Can you work these out from the model? Positions are in its coordinate system, mm. Round coordinates to 2 decimals unless told otherwise and drop trailing zeros. Loops run counter-clockwise (first coordinate to the right, second up) from the corner with the lowest first, then second, coordinate; pieces in that order, holes last.
(1) I want a section at B-B on y = 152.4. Write out the boundary of the cut face in (x, z).
(2) Will this pin go through, and if not, where does the flat tip stop? pin 1 Ø7 at (y, z) = (152.4, 69.85) entering from +X.
(3) I want a section at A-A on z = -139.7. Write out the boundary of the cut face in (x, y) (1 decimal).
(4) If I drill on line 1 along Y through (x, z) = (1.1, 69.85) (3 decimals); line 2 along Y through (x, z) = (3.85, 69) (3 decimals); line 3 along Z through (x, y) = (1.4, -152), over which ranges is the centre line in solid material (lowest first)?
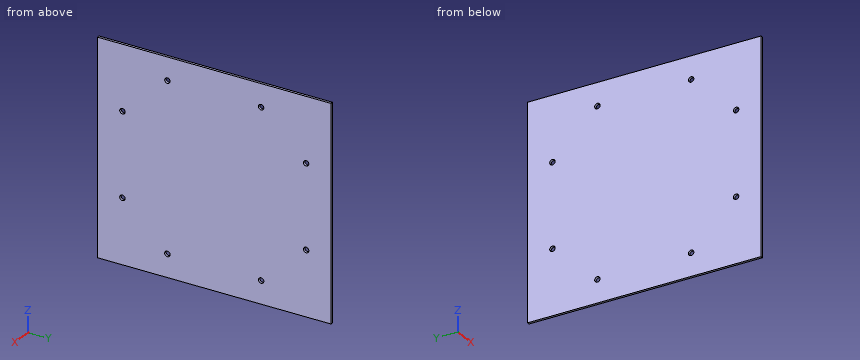
from build123d import *

# Parameters (mm, degrees)
SKETCH1_W            = 355.6
SKETCH1_H            = 387.35
SKETCH1_R            = 4.0005
BOSS_EXTRUDE1_DEPTH  = 4.064
M8_CLEARANCE_HOLE1_D = 9


with BuildPart() as part:
    # Sketch1 → Boss-Extrude1 (new body)
    # profile 1 of 9: a face of its own
    with BuildSketch(Plane(origin=(0, 0, 0), x_dir=(0, 0, -1), z_dir=(1, 0, 0))):
        Rectangle(SKETCH1_W, SKETCH1_H)
        with Locations((139.7, 77.7875)):
            Circle(SKETCH1_R, mode=Mode.SUBTRACT)
        with Locations((69.85, 152.4)):
            Circle(SKETCH1_R, mode=Mode.SUBTRACT)
        with Locations((-139.7, 77.7875)):
            Circle(SKETCH1_R, mode=Mode.SUBTRACT)
        with Locations((-139.7, -77.7875)):
            Circle(SKETCH1_R, mode=Mode.SUBTRACT)
        with Locations((-69.85, -152.4)):
            Circle(SKETCH1_R, mode=Mode.SUBTRACT)
        with Locations((69.85, -152.4)):
            Circle(SKETCH1_R, mode=Mode.SUBTRACT)
        with Locations((-69.85, 152.4)):
            Circle(SKETCH1_R, mode=Mode.SUBTRACT)
        with Locations((139.7, -77.7875)):
            Circle(SKETCH1_R, mode=Mode.SUBTRACT)
    # profile 2 of 9: a face of its own
    with BuildSketch(Plane(origin=(0, 0, 0), x_dir=(0, 0, -1), z_dir=(1, 0, 0))):
        with Locations((-69.85, -152.4)):
            Circle(SKETCH1_R)
    # profile 3 of 9: a face of its own
    with BuildSketch(Plane(origin=(0, 0, 0), x_dir=(0, 0, -1), z_dir=(1, 0, 0))):
        with Locations((69.85, -152.4)):
            Circle(SKETCH1_R)
    # profile 4 of 9: a face of its own
    with BuildSketch(Plane(origin=(0, 0, 0), x_dir=(0, 0, -1), z_dir=(1, 0, 0))):
        with Locations((139.7, -77.7875)):
            Circle(SKETCH1_R)
    # profile 5 of 9: a face of its own
    with BuildSketch(Plane(origin=(0, 0, 0), x_dir=(0, 0, -1), z_dir=(1, 0, 0))):
        with Locations((139.7, 77.7875)):
            Circle(SKETCH1_R)
    # profile 6 of 9: a face of its own
    with BuildSketch(Plane(origin=(0, 0, 0), x_dir=(0, 0, -1), z_dir=(1, 0, 0))):
        with Locations((69.85, 152.4)):
            Circle(SKETCH1_R)
    # profile 7 of 9: a face of its own
    with BuildSketch(Plane(origin=(0, 0, 0), x_dir=(0, 0, -1), z_dir=(1, 0, 0))):
        with Locations((-69.85, 152.4)):
            Circle(SKETCH1_R)
    # profile 8 of 9: a face of its own
    with BuildSketch(Plane(origin=(0, 0, 0), x_dir=(0, 0, -1), z_dir=(1, 0, 0))):
        with Locations((-139.7, 77.7875)):
            Circle(SKETCH1_R)
    # profile 9 of 9: a face of its own
    with BuildSketch(Plane(origin=(0, 0, 0), x_dir=(0, 0, -1), z_dir=(1, 0, 0))):
        with Locations((-139.7, -77.7875)):
            Circle(SKETCH1_R)
    extrude(amount=BOSS_EXTRUDE1_DEPTH)

    # M8 Clearance Hole1 (through all)
    with Locations(Plane(origin=(4.064, 0, 0), x_dir=(0, 0, -1), z_dir=(1, 0, 0))):
        with Locations((-139.7, 77.7875), (-69.85, 152.4), (69.85, 152.4), (139.7, 77.7875), (139.7, -77.7875), (69.85, -152.4), (-69.85, -152.4), (-139.7, -77.7875)):
            Hole(M8_CLEARANCE_HOLE1_D / 2)


solid = part.part
Filled sheet:
1. outline: (0, -177.8) - (4.06, -177.8) - (4.06, -74.35) - (0, -74.35) - close; (0, -65.35) - (4.06, -65.35) - (4.06, 65.35) - (0, 65.35) - close; (0, 74.35) - (4.06, 74.35) - (4.06, 177.8) - (0, 177.8) - close
2. pin 1: passes through
3. outline: (0, -193.7) - (4.1, -193.7) - (4.1, -82.3) - (0, -82.3) - close; (0, -73.3) - (4.1, -73.3) - (4.1, 73.3) - (0, 73.3) - close; (0, 82.3) - (4.1, 82.3) - (4.1, 193.7) - (0, 193.7) - close
4. line 1: y = -193.675 to -156.9, -147.9 to 147.9, 156.9 to 193.675
4. line 2: y = -193.675 to -156.819, -147.981 to 147.981, 156.819 to 193.675
4. line 3: z = -177.8 to -74.33, -65.37 to 65.37, 74.33 to 177.8
